```python
from build123d import *

# Parameters (mm, degrees)
SKETCH1_W                = 141
SKETCH1_H                = 12
BOSS_EXTRUDE1_DEPTH      = 1.5
SKETCH2_W                = 30
SKETCH2_H                = 3
SKETCH2_W_2              = 17
BOSS_EXTRUDE2_DEPTH      = 1.5
SKETCH12_W               = 25
SKETCH12_H               = 3
BOSS_EXTRUDE3_DEPTH      = 1.5
CUT_EXTRUDE8_DEPTH       = 2.5
CUT_EXTRUDE8_DEPTH_BACK  = 2.5
SKETCH13_W               = 35
SKETCH13_H               = 3
BOSS_EXTRUDE4_DEPTH      = 1.5
SKETCH15_W               = 11
SKETCH15_H               = 9
CUT_EXTRUDE10_DEPTH      = 2.5
CUT_EXTRUDE10_DEPTH_BACK = 2.5
FILLET4_R                = 3
CUT_EXTRUDE11_DEPTH      = 2.5
CUT_EXTRUDE11_DEPTH_BACK = 2.5
SKETCH17_W               = 3
SKETCH17_H               = 6
CUT_EXTRUDE12_DEPTH      = 2.5
CUT_EXTRUDE12_DEPTH_BACK = 2.5


with BuildPart() as part:
    # Sketch1 → Boss-Extrude1 (new body, symmetric)
    with BuildSketch(Plane(origin=(0, 0, 0), x_dir=(1, 0, 0), z_dir=(0, 1, 0))):
        Rectangle(SKETCH1_W, SKETCH1_H)
    extrude(amount=BOSS_EXTRUDE1_DEPTH, both=True)

    # Sketch2 → Boss-Extrude2 (add, symmetric)
    with BuildSketch(Plane(origin=(0, 0, 0), x_dir=(1, 0, 0), z_dir=(0, 1, 0))):
        with Locations((15.5, -7.5)):
            Rectangle(SKETCH2_W, SKETCH2_H)
        with Locations((62, -7.5)):
            Rectangle(SKETCH2_W_2, SKETCH2_H)
    extrude(amount=BOSS_EXTRUDE2_DEPTH, both=True)

    # Sketch12 → Boss-Extrude3 (add, symmetric)
    with BuildSketch(Plane(origin=(0, 0, 0), x_dir=(1, 0, 0), z_dir=(0, 1, 0))):
        with Locations((-38, -7.5)):
            Rectangle(SKETCH12_W, SKETCH12_H)
    extrude(amount=BOSS_EXTRUDE3_DEPTH, both=True)

    # Sketch11 → Cut-Extrude8 (cut, two sides)
    with BuildSketch(Plane(origin=(0, 0, 0), x_dir=(1, 0, 0), z_dir=(0, 1, 0))) as cut_extrude8_sk:
        with BuildLine():
            Line((-39.5, -2.73), (-39.5, 0))
            ThreePointArc((-39.5, 0), (-39.207106781, 0.707106781), (-38.5, 1))
            Line((-38.5, 1), (-37.5, 1))
            ThreePointArc((-37.5, 1), (-36.792893219, 0.707106781), (-36.5, 0))
            Line((-36.5, 0), (-36.5, -2.73))
            Line((-36.5, -2.73), (-35.15, -2.73))
            Line((-35.15, -2.73), (-35.15, -5))
            Line((-35.15, -5), (-36.5, -5))
            Line((-36.5, -5), (-36.5, -9))
            Line((-36.5, -9), (-39.5, -9))
            Line((-39.5, -9), (-39.5, -5))
            Line((-39.5, -5), (-40.85, -5))
            Line((-40.85, -5), (-40.85, -2.73))
            Line((-40.85, -2.73), (-39.5, -2.73))
        make_face()
        with BuildLine():
            Line((14, -9), (17, -9))
            Line((17, -9), (17, -5))
            Line((17, -5), (18.35, -5))
            Line((18.35, -5), (18.35, -2.73))
            Line((18.35, -2.73), (17, -2.73))
            Line((17, -2.73), (17, 0))
            ThreePointArc((17, 0), (16.707106781, 0.707106781), (16, 1))
            Line((16, 1), (15, 1))
            ThreePointArc((15, 1), (14.292893219, 0.707106781), (14, 0))
            Line((14, 0), (14, -2.73))
            Line((14, -2.73), (12.65, -2.73))
            Line((12.65, -2.73), (12.65, -5))
            Line((12.65, -5), (14, -5))
            Line((14, -5), (14, -9))
        make_face()
    extrude(amount=CUT_EXTRUDE8_DEPTH, mode=Mode.SUBTRACT)
    extrude(cut_extrude8_sk.sketch, amount=-CUT_EXTRUDE8_DEPTH_BACK, mode=Mode.SUBTRACT)

    # Sketch13 → Boss-Extrude4 (add, symmetric)
    with BuildSketch(Plane(origin=(0, 0, 0), x_dir=(1, 0, 0), z_dir=(0, 1, 0))):
        with Locations((-28, 7.5)):
            Rectangle(SKETCH13_W, SKETCH13_H)
        with Locations((28, 7.5)):
            Rectangle(SKETCH13_W, SKETCH13_H)
    extrude(amount=BOSS_EXTRUDE4_DEPTH, both=True)

    # Sketch15 → Cut-Extrude10 (cut, two sides)
    with BuildSketch(Plane(origin=(0, 0, 0), x_dir=(1, 0, 0), z_dir=(0, 1, 0))) as cut_extrude10_sk:
        with Locations((62, -0.5)):
            Rectangle(SKETCH15_W, SKETCH15_H)
    extrude(amount=CUT_EXTRUDE10_DEPTH, mode=Mode.SUBTRACT)
    extrude(cut_extrude10_sk.sketch, amount=-CUT_EXTRUDE10_DEPTH_BACK, mode=Mode.SUBTRACT)

    # Fillet4
    fillet4_edges = [part.edges().sort_by_distance(p)[0] for p in [
        (56.5, 0, 5),
        (56.5, 0, -4),
        (67.5, 0, -4),
        (67.5, 0, 5),
    ]]
    fillet(fillet4_edges, radius=FILLET4_R)

    # Sketch16 → Cut-Extrude11 (cut, two sides)
    with BuildSketch(Plane(origin=(0, 0, 0), x_dir=(1, 0, 0), z_dir=(0, 1, 0))) as cut_extrude11_sk:
        Polygon((53.5, 0), (51.25, 1.299038106), (51.25, -1.299038106), align=None)
    extrude(amount=CUT_EXTRUDE11_DEPTH, mode=Mode.SUBTRACT)
    extrude(cut_extrude11_sk.sketch, amount=-CUT_EXTRUDE11_DEPTH_BACK, mode=Mode.SUBTRACT)

    # Sketch17 → Cut-Extrude12 (cut, two sides)
    with BuildSketch(Plane(origin=(0, 0, 0), x_dir=(1, 0, 0), z_dir=(0, 1, 0))) as cut_extrude12_sk:
        with Locations((-69, 0)):
            Rectangle(SKETCH17_W, SKETCH17_H)
    extrude(amount=CUT_EXTRUDE12_DEPTH, mode=Mode.SUBTRACT)
    extrude(cut_extrude12_sk.sketch, amount=-CUT_EXTRUDE12_DEPTH_BACK, mode=Mode.SUBTRACT)


solid = part.part
```
The model under review builds one solid part; all positions refer to its coordinate system, in mm. A direction names the side the tool comes from. Round coordinates to 2 decimals unless told otherwise and drop trailing zeros. Order: outer loops, then holes, each group sorted by start corner. A loop starts at its lowest first (then second) coordinate and runs counter-clockwise, first axis right, second up. Notation, with made-up numbers: M 42,4 L 64,4 A7 ccw 64,10 Z; hole C 32.5,-30.5 d3. An arc over 180 degrees is marked long. Use a Markdown table: item, result.
1) Tool access review of faces 5 (the face through (-10.5, 0, -7)), 6 (the face through (-35.15, 0, 4)), 7 (the face through (-58, 0, -6)), 8 (the face through (-39.5, 0, 7)), 9 (the face through (-61, 0, 6)): name each direction out of +Z, -Z, +X, -X, +Y, -Y from which nothing blocks a thin tool from reaching the whole face with its end or side.
Report:
| item | result |
|---|---|
| face 5 | -Z, +Y, -Y |
| face 6 | +Y, -Y |
| face 7 | -Z, -X, +Y, -Y |
| face 8 | +Z, +Y, -Y |
| face 9 | +Z, -X, +Y, -Y |
2) Consider section B-B (y = -1). Give the number of separate pieces and of enclosed holes in the cut face, then the cut area to 3 significant figures.
Report:
| item | result |
|---|---|
| separate pieces | 1 |
| enclosed holes | 2 |
| area | 1,930 mm^2 |
3) Consider section A-A (x = -17.5). Write out the cut boundary in (y, z), then the cut area to 3 significant figures.
Report:
| item | result |
|---|---|
| outline | M -1.5,-9 L 1.5,-9 L 1.5,6 L -1.5,6 Z |
| area | 45.0 mm^2 |
4) Wall thickness on line 1 along X through (y, z) = (0.7, 7.5); line 2 along X through (y, z) = (1.1, 5.75); line 3 along X through (y, z) = (0.85, -0.5): over which ranges is each line inside the solid? List them lowest first. Write a range as [from, to].
Report:
| item | result |
|---|---|
| line 1 | [-50.5, -39.5], [-36.5, -25.5], [0.5, 14], [17, 30.5], [53.5, 70.5] |
| line 2 | [-70.5, -39.5], [-36.5, 14], [17, 70.5] |
| line 3 | [-67.5, -39.37], [-36.63, 14.13], [16.87, 51.25], [52.63, 56.5], [67.5, 70.5] |
5) Draft analysis for pull direction Z (two halves, no side actions). For faces 1 (the face through (52.36, -0.02, 0.66)), 2 (the face through (0.5, 0, 8)), 3 (the face through (-67.5, 0, 0)), 4 (the face through (28, 0, -9)), state which applies: released by +Z, released by -Z, zero draft, split by the parting line, or undercut.
Report:
| item | result |
|---|---|
| face 1 | undercut |
| face 2 | zero draft |
| face 3 | undercut |
| face 4 | released by -Z |
6) Insertion check: pin 1 (0.9 mm diameter, centred on x = -6.5, y = 0.5, fed in from +Z); pin 2 (1.5 mm diameter, centred on x = 61, y = 0.5, fed in from -Z). Each pin has a flat end and moves straight along its axis. Give the tip position at first contact, or say it passes through.
Report:
| item | result |
|---|---|
| pin 1 | z = 6 |
| pin 2 | z = -6 |
